Source: CAD feature listing. Evaluate the final solid. Frame: model axes, mm. A direction names the side the tool comes from. Coordinates: 2 decimals unless noted, no trailing zeros. Order: outer loops, then holes, each group sorted by start corner. A loop starts at its lowest first (then second) coordinate and runs counter-clockwise, first axis right, second up.
Item 1: Section D-D on z = 4.5. Return the cut outline in (x, y).
Item 2: Contact query for flat-ended pins moving along their axis: P1, Ø1.3, axis at x = 50, y = 7.5, coming from the -Z side; P2, Ø4, axis at y = -13.5, z = 14, coming from the +X side; P3, Ø4, axis at x = 33.5, z = -4, coming from the +Y side; P4, Ø3.5, axis at x = 22, y = 20.5, coming from the -Z side. Output: stop coordinate, or through.
Item 3: Reachability of faces 1 (the flat face through (23, -19, 3)), 2 (the flat face through (48, -7, -8)), 3 (the cylindrical face through (-6.91, -3.57, -8.2)), 4 (the flat face through (3.75, 7, -8)), 5 (the flat face through (5, -11.094, -14)) from +Z, -Z, +X, -X, +Y, -Y: full face, straight path, thin tool, end or side. Return the list, or none.
Item 4: Mould query, pull axis X, two halves, no side actions, for faces 6 (the flat face through (11.25, -16, -14)), 7 (the flat face through (11, -13, 7)), 8 (the flat face through (3, -16, -11.5)). Classes: released by +X, released by -X, zero draft, split by the parting line, or undercut.
Item 5: Section C-C on x = 16. Return the cut outline in (y, z).
Item 6: Section A-A on x = 50. Return the cut outline in (y, z), then the cut area to 3 significant figures.
Item 7: Ray query, line 1 (Y direction, x = -7.5, z = -9); line 2 (Z direction, x = 22.5, y = 20.5); line 3 (Y direction, x = 16, z = -2). Return the intervals inside material, ascending.
Item 8: Section B-B on y = -23. Return the cut outline in (x, z), then the cut area to 3 significant figures.
from build123d import *

# Parameters (mm, degrees)
SKETCH009_R     = 3
SKETCH009_R_2   = 1.1
PAD004_DEPTH    = 6.5
PAD005_DEPTH    = 5
SKETCH017_W     = 3
SKETCH017_H     = 10
SKETCH017_H_2   = 15
PAD010_DEPTH    = 8
SKETCH018_R     = 3
PAD011_DEPTH    = 24
SKETCH019_R     = 1.2
POCKET004_DEPTH = 3
SKETCH020_R     = 1.2
POCKET005_DEPTH = 3


with BuildPart() as part:
    # Sketch009 → Pad004 (new body)
    with BuildSketch(Plane.XY.offset(-5)):
        with BuildLine():
            Line((42.5, 10), (52.5, 10))
            Line((52.5, 10), (52.5, -7))
            Line((52.5, -7), (42.5, -7))
            Line((42.5, -7), (42.5, -15))
            Line((42.5, -15), (21, -15))
            ThreePointArc((11, -15), (16, -20), (21, -15))
            Line((0, -15), (11, -15))
            Line((0, -7), (0, -15))
            Line((-10, -7), (0, -7))
            Line((-10, 10), (-10, -7))
            Line((0, 10), (-10, 10))
            Line((0, 10), (0, 18))
            Line((0, 18), (42.5, 18))
            Line((42.5, 18), (42.5, 10))
        make_face()
        with Locations((16, -15)):
            Circle(SKETCH009_R, mode=Mode.SUBTRACT)
        with Locations((-7.5, -4.5)):
            Circle(SKETCH009_R_2, mode=Mode.SUBTRACT)
        with Locations((-7.5, 7.5)):
            Circle(SKETCH009_R_2, mode=Mode.SUBTRACT)
        with Locations((50, 7.5)):
            Circle(SKETCH009_R_2, mode=Mode.SUBTRACT)
        with Locations((50, -4.5)):
            Circle(SKETCH009_R_2, mode=Mode.SUBTRACT)
        with Locations((7.5, -4.5)):
            Circle(SKETCH009_R_2, mode=Mode.SUBTRACT)
        with Locations((35, -4.5)):
            Circle(SKETCH009_R_2, mode=Mode.SUBTRACT)
        Polygon((38.75, 14.5), (38.75, 0.5), (32.75, 0.5), (32.75, -11.5), (9.75, -11.5), (9.75, 0.5), (3.75, 0.5), (3.75, 14.5), align=None, mode=Mode.SUBTRACT)
    extrude(amount=-PAD004_DEPTH)

    # Sketch010 → Pad005 (new body)
    with BuildSketch(Plane(origin=(0, 0, -11.5), x_dir=(1, 0, 0), z_dir=(0, 0, -1))):
        with BuildLine():
            Line((11.25, 20.094157), (11.25, 11.094157))
            Line((11.25, 11.094157), (-2.172983, 11.094157))
            ThreePointArc((-2.172983, 11.094157), (16, -33.5), (34.172983, 11.094157))
            Line((34.172983, 11.094157), (20.75, 11.094157))
            Line((20.75, 11.094157), (20.75, 20.094157))
            ThreePointArc((20.75, 20.094157), (16, -35.5), (11.25, 20.094157))
        make_face()
    extrude(amount=PAD005_DEPTH)

    # Sketch017 → Pad010 (new body)
    with BuildSketch(Plane.XY.offset(-5)):
        with Locations((22.75, 19.5)):
            Rectangle(SKETCH017_W, SKETCH017_H)
        with Locations((22.75, -19)):
            Rectangle(SKETCH017_W, SKETCH017_H_2)
    extrude(amount=PAD010_DEPTH)

    # Sketch018 → Pad011 (new body)
    with BuildSketch(Plane.XY.offset(-5)):
        with BuildLine():
            ThreePointArc((11, -15), (16, -20), (21, -15))
            Line((21.25, -15), (21, -15))
            Line((21.25, -11.5), (21.25, -15))
            Line((11, -11.5), (21.25, -11.5))
            Line((11, -15), (11, -11.5))
        make_face()
        with Locations((16, -15)):
            Circle(SKETCH018_R, mode=Mode.SUBTRACT)
    extrude(amount=PAD011_DEPTH)

    # Sketch019 → Pocket004 (cut)
    with BuildSketch(Plane(origin=(21.25, 0, -5), x_dir=(0, -1, 0), z_dir=(-1, 0, 0))):
        with Locations((23, 3.757359)):
            Circle(SKETCH019_R)
    extrude(amount=-POCKET004_DEPTH, mode=Mode.SUBTRACT)

    # Sketch020 → Pocket005 (cut)
    with BuildSketch(Plane(origin=(21.25, 0, -5), x_dir=(0, -1, 0), z_dir=(-1, 0, 0))):
        with Locations((-20.5, 4.225083)):
            Circle(SKETCH020_R)
    extrude(amount=-POCKET005_DEPTH, mode=Mode.SUBTRACT)


solid = part.part
Answer list:
1. outline: (11, -15) arc R5 ccw to (21, -15) - (21.25, -15) - (21.25, -11.5) - (11, -11.5) - close; hole circle Ø6 at (16, -15)
2. P1: passes through
2. P2: stops at x = 21.25
2. P3: stops at y = 18
2. P4: stops at z = -5
3. face 1: +Z, +X, +Y, -Y
3. face 2: +Z, -Z, +X, -Y
3. face 3: +Z
3. face 4: +Z, -Z
3. face 5: -Z
4. face 6: undercut
4. face 7: released by -X
4. face 8: zero draft
5. outline: (-20, -11.5) - (-18, -11.5) - (-18, 19) - (-20, 19) - close; (-12, -11.5) - (-11.5, -11.5) - (-11.5, 19) - (-12, 19) - close; (14.5, -11.5) - (18, -11.5) - (18, -5) - (14.5, -5) - close; (33.5, -16.5) - (35.5, -16.5) - (35.5, -11.5) - (33.5, -11.5) - close
6. outline: (-7, -11.5) - (-5.6, -11.5) - (-5.6, -5) - (-7, -5) - close; (-3.4, -11.5) - (6.4, -11.5) - (6.4, -5) - (-3.4, -5) - close; (8.6, -11.5) - (10, -11.5) - (10, -5) - (8.6, -5) - close
6. area: 81.9 mm2
7. line 1: y = -7 to -5.6, -3.4 to 6.4, 8.6 to 10
7. line 2: z = -5 to -1.97, 0.43 to 3
7. line 3: y = -20 to -18, -12 to -11.5
8. outline: (21.25, -5) - (24.25, -5) - (24.25, -2.44) - (21.25, -2.44) - close; (21.25, -0.04) - (24.25, -0.04) - (24.25, 3) - (21.25, 3) - close
8. area: 16.8 mm2
